Here's how the part is built. I have some questions about the finished solid (model axes, mm). A direction names the side the tool comes from. Round coordinates to 2 decimals unless told otherwise and drop trailing zeros. Loops run counter-clockwise (first coordinate to the right, second up) from the corner with the lowest first, then second, coordinate; pieces in that order, holes last. Notation, with made-up numbers: M 63,53 L 69,53 A30 ccw 69,78 Z; hole C 38,28.25 d10. An arc over 180 degrees is marked long. Write each question's results on one line, items separated by ' | '. Start each with the question number.
```python
from build123d import *

# Parameters (mm, degrees)
SKETCH_1_R      = 5
SKETCH_1_R_2    = 2.1
SKETCH_1_R_3    = 1.6
SKETCH_1_R_4    = 12.5
EXTRUDE_1_DEPTH = 3
FILLET_1_R      = 10
FILLET_2_R      = 10


with BuildPart() as part:
    # 草图1 → 凸台-拉伸1 (new body)
    with BuildSketch(Plane.XY):
        with BuildLine():
            Line((12.419223494, -15.676826458), (153.603692908, -23.133474126))
            ThreePointArc((153.603692908, -23.133474126), (157.711237696, -22.783135564), (161.568286957, -21.32785817))
            Line((161.568286957, -21.32785817), (192.671157578, -4.391169028))
            ThreePointArc((192.671157578, -4.391169028), (195.155704471, 1.10792866), (190.538680801, 4.993303941))
            Line((190.538680801, 4.993303941), (155.185935535, 6.824771956))
            Line((155.185935535, 6.824771956), (14.001466121, 14.281419623))
            ThreePointArc((14.001466121, 14.281419623), (-19.972164054, 1.054828418), (12.419223494, -15.676826458))
        make_face()
        with Locations((154.394814221, -8.154351085)):
            Circle(SKETCH_1_R, mode=Mode.SUBTRACT)
        with Locations((190.28, 0)):
            Circle(SKETCH_1_R_2, mode=Mode.SUBTRACT)
        with Locations((0, 16)):
            Circle(SKETCH_1_R_3, mode=Mode.SUBTRACT)
        Circle(SKETCH_1_R_4, mode=Mode.SUBTRACT)
        with Locations((13.856406461, -8)):
            Circle(SKETCH_1_R_3, mode=Mode.SUBTRACT)
        with Locations((-13.856406461, -8)):
            Circle(SKETCH_1_R_3, mode=Mode.SUBTRACT)
    extrude(amount=EXTRUDE_1_DEPTH)

    # 圆角1
    fillet_1_edges = [part.edges().sort_by_distance(p)[0] for p in [
        (14.001466121, 14.281419623, 1.5),
    ]]
    fillet(fillet_1_edges, radius=FILLET_1_R)

    # 圆角2
    fillet_2_edges = [part.edges().sort_by_distance(p)[0] for p in [
        (12.419223494, -15.676826458, 1.5),
    ]]
    fillet(fillet_2_edges, radius=FILLET_2_R)


solid = part.part
```
Item 1: If we section it at D-D on x = 170: Please give me the cut outline in (y, z).
Item 2: Which directions (+Z, -Z, +X, -X, +Y, -Y) give clear straight access to the entire face, cutting with the end or side of a thin tool? Please do faces 1 (the face through (83.721, -19.443, 1.479)), 2 (the face through (195.175, 1.019, 1.479)).
Item 3: If we section it at C-C on x = 73: Please give me the cut outline in (y, z), and give its area (3 significant figures).
Item 4: I need wall thicknesses on L1, parallel to Y at x = 0, z = 1.8; L2, parallel to X at y = -4, z = 1.8; L3, parallel to X at y = -11.5, z = 1.25. Which ranges of each line are inside material? Lowest first, please.
Item 5: If we section it at A-A on y = 0: Please give me the cut outline in (x, z), and give its area (3 significant figures).
Item 6: I'm going to push a flat-ended pin straight in: pin 1 (20 mm diameter, centred on x = 0, y = 0, fed in from -Z). Where does the tip first touch, or does it pass through?
Item 7: If we section it at B-B on z = 2.2: Please give me the cut outline in (x, y).
Item 8: If we mould it in two halves opening along X, with no side actions, what happens to faces 3 (the face through (149.4, -7.9, 1.5)), 4 (the face through (176.9, -12.98, 1.48)), 5 (the face through (86, -6, 0))? For each: released by +X, released by -X, zero draft, split by the parting line, or undercut.
Numbers:
1) outline: M -16.74,0 L 6.06,0 L 6.06,3 L -16.74,3 Z
2) face 1: +Z, -Z, -Y | face 2: +Z, -Z, +X
3) outline: M -18.88,0 L 11.17,0 L 11.17,3 L -18.88,3 Z | area: 90.1 mm²
4) L1: -20 to -12.5, 12.5 to 14.4, 17.6 to 20 | L2: -19.6 to -11.84, 11.84 to 151.61, 157.18 to 193.28 | L3: -16.36 to -4.9, 4.9 to 150.68, 158.11 to 179.62
5) outline: M -20,0 L -12.5,0 L -12.5,3 L -20,3 Z; M 12.5,0 L 188.18,0 L 188.18,3 L 12.5,3 Z; M 192.38,0 L 195.28,0 L 195.28,3 L 192.38,3 Z | area: 558 mm²
6) pin 1: through
7) outline: M 10.16,-17.23 A10 cw 15.77,-15.85 L 153.6,-23.13 A15 ccw 161.57,-21.33 L 192.67,-4.39 A5 ccw 190.54,4.99 L 155.19,6.82 L 17.35,14.1 A10 cw 11.92,16.06 A20 ccw long Z; hole C -13.86,-8 d3.2; hole C 0,0 d25; hole C 0,16 d3.2; hole C 13.86,-8 d3.2; hole C 154.39,-8.15 d10; hole C 190.28,0 d4.2
8) face 3: undercut | face 4: released by +X | face 5: zero draft
